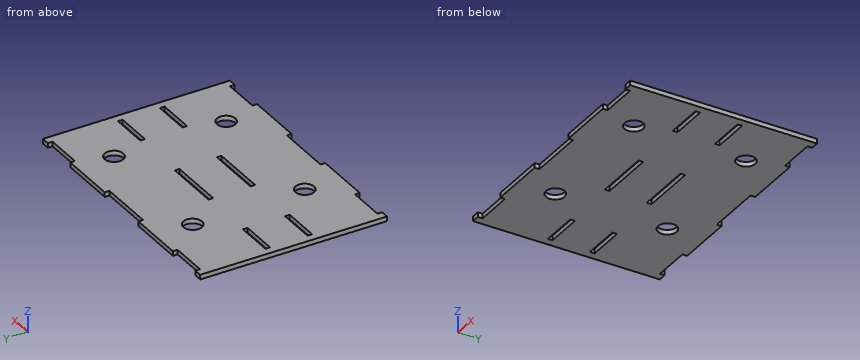
from build123d import *

# Parameters (mm, degrees)
F0_R     = 6.35
F0_W     = 25.4
F0_H     = 3.175
F0_W_2   = 38.1
F1_DEPTH = 3.175


# Not quite as in the source:
# - a feature names something its author has since deleted; it is built from what else it names


with BuildPart() as f1:
    # F0 (on Top) → F1 (new body)
    with BuildSketch(Plane.XY):
        Polygon((-70.7512, 63.5), (-76.2, 63.5), (-76.2, -63.5), (-70.7512, -63.5), (-70.7512, -60.325), (-45.3512, -60.325), (-45.3512, -63.5), (-6.35, -63.5), (-6.35, -60.325), (31.75, -60.325), (31.75, -63.5), (70.7512, -63.5), (70.7512, -60.325), (96.1512, -60.325), (96.1512, -63.5), (101.6, -63.5), (101.6, 63.5), (96.1512, 63.5), (96.1512, 60.325), (70.7512, 60.325), (70.7512, 63.5), (31.75, 63.5), (31.75, 60.325), (-6.35, 60.325), (-6.35, 63.5), (-45.3512, 63.5), (-45.3512, 60.325), (-70.7512, 60.325), align=None)
        with Locations((-25.4, -38.1)):
            Circle(F0_R, mode=Mode.SUBTRACT)
        with Locations((-58.0512, -14.2875)):
            Rectangle(F0_W, F0_H, mode=Mode.SUBTRACT)
        with Locations((63.5, -38.1)):
            Circle(F0_R, mode=Mode.SUBTRACT)
        with Locations((12.7, -14.2875)):
            Rectangle(F0_W_2, F0_H, mode=Mode.SUBTRACT)
        with Locations((83.4512, -14.2875)):
            Rectangle(F0_W, F0_H, mode=Mode.SUBTRACT)
        with Locations((-58.0512, 14.2875)):
            Rectangle(F0_W, F0_H, mode=Mode.SUBTRACT)
        with Locations((-25.4, 38.1)):
            Circle(F0_R, mode=Mode.SUBTRACT)
        with Locations((12.7, 14.2875)):
            Rectangle(F0_W_2, F0_H, mode=Mode.SUBTRACT)
        with Locations((83.4512, 14.2875)):
            Rectangle(F0_W, F0_H, mode=Mode.SUBTRACT)
        with Locations((63.5, 38.1)):
            Circle(F0_R, mode=Mode.SUBTRACT)
    extrude(amount=F1_DEPTH)


solid = f1.part
Source: CAD feature listing. Evaluate the final solid. Frame: model axes, mm. Give positions to 0.01 mm unless a question says otherwise; leave off trailing zeros. Write each loop counter-clockwise with the first axis right and the second up, starting at its lowest first coordinate (ties: lowest second). Pieces come first, ordered by that corner, then holes. Notation, with made-up numbers: (-34.75, 63) - (13.25, 63) arc R12 cw to (13.25, 73) - close; hole circle Ø8 at (-24.75, -32). An arc over 180 degrees is marked (long way). Write item = value, one per line. Start each with the question number.
Q1. Cut plane C-C, the plane z = 1.4. Give the number of separate pieces and of enclosed holes in the cut face, then the cut area to 3 significant figures.
Q2. Cut plane A-A, the plane x = 63.5. Return loops of the section in (y, z) (3 decimals), then the cut area to 3 significant figures.
Q3. Cut plane B-B, the plane y = 38.1. Return loops of the section in (x, z) (3 decimals).
Q4. Pin query (flat end, axial travel): pin 1 Ø1 at (x, z) = (85.5, 1) entering from -Y (3 decimals); pin 2 Ø1.6 at (x, z) = (78.5, 2.5) entering from +Y (3 decimals). Return the tip coordinate at first contact, or that it passes through.
Q5. Material intervals for probe 1 along Y at (x, z) = (91.5, 1.7) (3 decimals); probe 2 along X at (y, z) = (33, 2.85); probe 3 along X at (y, z) = (35, 2.4), sorted ascending.
Computed values:
q1.separate_pieces = 1
q1.enclosed_holes = 10
q1.area = 20,900 mm²
q2.outline = (-63.5, 0) - (-44.45, 0) - (-44.45, 3.175) - (-63.5, 3.175) - close; (-31.75, 0) - (31.75, 0) - (31.75, 3.175) - (-31.75, 3.175) - close; (44.45, 0) - (63.5, 0) - (63.5, 3.175) - (44.45, 3.175) - close
q2.area = 323 mm²
q3.outline = (-76.2, 0) - (-31.75, 0) - (-31.75, 3.175) - (-76.2, 3.175) - close; (-19.05, 0) - (57.15, 0) - (57.15, 3.175) - (-19.05, 3.175) - close; (69.85, 0) - (101.6, 0) - (101.6, 3.175) - (69.85, 3.175) - close
q4.pin_1 = -60.325
q4.pin_2 = 60.325
q5.probe_1 = -60.325 to -15.875, -12.7 to 12.7, 15.875 to 60.325
q5.probe_2 = -76.2 to -29.18, -21.62 to 59.72, 67.28 to 101.6
q5.probe_3 = -76.2 to -30.94, -19.86 to 57.96, 69.04 to 101.6
